from build123d import *

# Parameters (mm, degrees)
F1_DEPTH = 660.4
F3_DEPTH = 49.2135
F2_W     = 30.1752
F2_H     = 101.6
F2_R     = 3.175
F4_DEPTH = 3.175
F5_D     = 6.35
F6_D     = 9.525


with BuildPart() as f1:
    # F0 (on Front) → F1 (new body, symmetric)
    with BuildSketch(Plane.XZ):
        Polygon((23.312041, 26.91088), (-25.900459, 26.91088), (-25.900459, -22.30162), (-19.550459, -22.30162), (-19.550459, 20.56088), (23.312041, 20.56088), align=None)
    extrude(amount=F1_DEPTH, both=True)

    # F2 (on face) → F3 (cut, through all)
    with BuildSketch(Plane.XY.offset(26.91088)):
        Polygon((16.962041, 552.5516), (23.312041, 552.5516), (23.312041, 660.4), (16.962041, 660.4), (16.962041, 558.8), align=None)
        Polygon((23.312041, -660.4), (23.312041, -552.5516), (16.962041, -552.5516), (16.962041, -558.8), (16.962041, -660.4), align=None)
    extrude(amount=-F3_DEPTH, mode=Mode.SUBTRACT)

    # F2 (on face) → F4 (cut)
    with BuildSketch(Plane.XY.offset(26.91088)):
        with Locations((1.874441, -609.6)):
            Rectangle(F2_W, F2_H)
        with Locations((-3.688159, -647.7)):
            Circle(F2_R, mode=Mode.SUBTRACT)
        with Locations((-3.688159, -596.9)):
            Circle(F2_R, mode=Mode.SUBTRACT)
        with Locations((7.437041, -622.3)):
            Circle(F2_R, mode=Mode.SUBTRACT)
        with Locations((7.437041, -571.5)):
            Circle(F2_R, mode=Mode.SUBTRACT)
        with Locations((1.874441, 609.6)):
            Rectangle(F2_W, F2_H)
        with Locations((-3.688159, 571.5)):
            Circle(F2_R, mode=Mode.SUBTRACT)
        with Locations((-3.688159, 622.3)):
            Circle(F2_R, mode=Mode.SUBTRACT)
        with Locations((7.437041, 596.9)):
            Circle(F2_R, mode=Mode.SUBTRACT)
        with Locations((7.437041, 647.7)):
            Circle(F2_R, mode=Mode.SUBTRACT)
    extrude(amount=-F4_DEPTH, mode=Mode.SUBTRACT)

    # F5 (through all)
    with Locations(Plane.XY.offset(26.91088)):
        with Locations((-3.688159, -596.9), (7.437041, -571.5), (7.437041, -622.3), (-3.688159, -647.7), (7.437041, 596.9), (-3.688159, 622.3), (7.437041, 647.7), (-3.688159, 571.5)):
            Hole(F5_D / 2)

    # F6 (through all)
    with Locations(Plane.XY.offset(26.91088)):
        with Locations((0, -546.1), (0, 546.1)):
            Hole(F6_D / 2)


solid = f1.part
Input: part model. Units: mm. Frame: model coordinates. A direction names the side the tool comes from. Coordinates: 2 decimals unless noted, no trailing zeros. Loops run counter-clockwise (first coordinate to the right, second up) from the corner with the lowest first, then second, coordinate; pieces in that order, holes last. Notation, with made-up numbers: (9, -18) -> (55, -18) arc R26 cw to (55, 16) -> close; hole circle Ø6 at (77.25, -3). An arc over 180 degrees is marked (long way). Write item = value, one per line. Start each with the question number.
Item 1: Cut plane A-A, the plane y = -361.5. Return loops of the section in (x, z).
Item 2: First-contact query: P1, Ø3, axis at y = -494, z = -9, coming from the +X side; P2, Ø15, axis at x = -2.5, y = -607, coming from the +Z side; P3, Ø1.5, axis at x = 15.5, y = 137.5, coming from the -Z side; P4, Ø10, axis at y = -344, z = 19.5, coming from the +X side. Flat tips, straight axial feed; report the tip coordinate or a pass-through.
Item 3: Cut plane B-B, the plane z = -5. Return loops of the section in (x, y), plus the area to 3 significant figures.
Item 4: Material intervals for line 1 (Y direction, x = 0, z = 22.5); line 2 (X direction, y = -622.3, z = 21.7); line 3 (X direction, y = -174, z = 15), sorted ascending.
Item 5: Reachability of faces 1 (the face through (-20, -660.4, 8)), 2 (the face through (-19.55, -9, -1)), 3 (the face through (2, 610, 23.736)), 4 (the face through (2, -609, 23.736)), 5 (the face through (-1, -9, 26.911)) from +Z, -Z, +X, -X, +Y, -Y: full face, straight path, thin tool, end or side. Return the list, or none.
Ans:
q1.outline = (-25.9, -22.3) -> (-19.55, -22.3) -> (-19.55, 20.56) -> (23.31, 20.56) -> (23.31, 26.91) -> (-25.9, 26.91) -> close
q2.P1 = -19.55
q2.P2 = 23.74
q2.P3 = 20.56
q2.P4 = 23.31
q3.outline = (-25.9, -660.4) -> (-19.55, -660.4) -> (-19.55, 660.4) -> (-25.9, 660.4) -> close
q3.area = 8,390 mm²
q4.line_1 = -660.4 to -550.86, -541.34 to 541.34, 550.86 to 660.4
q4.line_2 = -25.9 to 4.26, 10.61 to 16.96
q4.line_3 = -25.9 to -19.55
q5.face_1 = +Z, -Z, +X, -X, -Y
q5.face_2 = -Z, +X, +Y, -Y
q5.face_3 = +Z, +X, +Y
q5.face_4 = +Z, +X, -Y
q5.face_5 = +Z, +X, -X, +Y, -Y
